Geometry: final body of the model. Coordinates: model frame, mm. Coordinates: 2 decimals unless noted, no trailing zeros. Write each loop counter-clockwise with the first axis right and the second up, starting at its lowest first coordinate (ties: lowest second). Pieces come first, ordered by that corner, then holes. Notation, with made-up numbers: (30, 3.25) - (66, 3.25) arc R33 ccw to (66, 40.25) - close; hole circle Ø11 at (-39.75, -13). An arc over 180 degrees is marked (long way). Put each result on its own line as item: value.
```python
from build123d import *

# Parameters (mm, degrees)
ESQUISSE1_W                = 381
ESQUISSE1_H                = 381
BOSS_EXTRU_1_DEPTH         = 6.35
ESQUISSE2_W                = 38.1
ESQUISSE2_H                = 6.35
BOSS_EXTRU_2_DEPTH         = 6.35
R_P_TITION_LIN_AIRE1_COUNT = 4
R_P_TITION_LIN_AIRE1_PITCH = 76.2
SYM_TRIE1_COPY_1_SKETCH_W  = 38.1
SYM_TRIE1_COPY_1_SKETCH_H  = 6.35
SYM_TRIE1_COPY_1_DEPTH     = 6.35
SYM_TRIE1_COPY_2_SKETCH_W  = 38.1
SYM_TRIE1_COPY_2_SKETCH_H  = 6.35
SYM_TRIE1_COPY_2_DEPTH     = 6.35
SYM_TRIE1_COPY_3_SKETCH_W  = 38.1
SYM_TRIE1_COPY_3_SKETCH_H  = 6.35
SYM_TRIE1_COPY_3_DEPTH     = 6.35
ESQUISSE3_W                = 38.1
ESQUISSE3_H                = 6.35
BOSS_EXTRU_3_DEPTH         = 6.35
R_P_TITION_LIN_AIRE2_COUNT = 4
R_P_TITION_LIN_AIRE2_PITCH = 76.2
SYM_TRIE2_COPY_1_SKETCH_W  = 38.1
SYM_TRIE2_COPY_1_SKETCH_H  = 6.35
SYM_TRIE2_COPY_1_DEPTH     = 6.35
SYM_TRIE2_COPY_2_SKETCH_W  = 38.1
SYM_TRIE2_COPY_2_SKETCH_H  = 6.35
SYM_TRIE2_COPY_2_DEPTH     = 6.35
SYM_TRIE2_COPY_3_SKETCH_W  = 38.1
SYM_TRIE2_COPY_3_SKETCH_H  = 6.35
SYM_TRIE2_COPY_3_DEPTH     = 6.35


with BuildPart() as part:
    # Esquisse1 → Boss.-Extru.1 (new body)
    with BuildSketch(Plane(origin=(0, 0, 0), x_dir=(1, 0, 0), z_dir=(0, 1, 0))):
        Rectangle(ESQUISSE1_W, ESQUISSE1_H)
    extrude(amount=BOSS_EXTRU_1_DEPTH)

    # Esquisse2 → Boss.-Extru.2 (add)
    with BuildSketch(Plane(origin=(190.5, 0, 0), x_dir=(0, 0, -1), z_dir=(1, 0, 0))):
        with Locations((-114.3, 3.175)):
            Rectangle(ESQUISSE2_W, ESQUISSE2_H)
    boss_extru_2 = extrude(amount=BOSS_EXTRU_2_DEPTH)

    # Répétition linéaire1: Boss.-Extru.2 ×4
    with Locations(*[(0, 0, -i * R_P_TITION_LIN_AIRE1_PITCH) for i in range(1, R_P_TITION_LIN_AIRE1_COUNT)]):
        add(boss_extru_2)

    # Symétrie1: Boss.-Extru.2 across plane
    add(boss_extru_2.mirror(Plane(origin=(0, 0, 0), x_dir=(0, 0, 1), z_dir=(1, 0, 0))))

    # Symétrie1 copy 1 sketch → Symétrie1 copy 1 (add)
    with BuildSketch(Plane(origin=(-190.5, 0, -76.2), x_dir=(0, 0, -1), z_dir=(-1, 0, 0))):
        with Locations((-114.3, -3.175)):
            Rectangle(SYM_TRIE1_COPY_1_SKETCH_W, SYM_TRIE1_COPY_1_SKETCH_H)
    extrude(amount=SYM_TRIE1_COPY_1_DEPTH)

    # Symétrie1 copy 2 sketch → Symétrie1 copy 2 (add)
    with BuildSketch(Plane(origin=(-190.5, 0, -152.4), x_dir=(0, 0, -1), z_dir=(-1, 0, 0))):
        with Locations((-114.3, -3.175)):
            Rectangle(SYM_TRIE1_COPY_2_SKETCH_W, SYM_TRIE1_COPY_2_SKETCH_H)
    extrude(amount=SYM_TRIE1_COPY_2_DEPTH)

    # Symétrie1 copy 3 sketch → Symétrie1 copy 3 (add)
    with BuildSketch(Plane(origin=(-190.5, 0, -228.6), x_dir=(0, 0, -1), z_dir=(-1, 0, 0))):
        with Locations((-114.3, -3.175)):
            Rectangle(SYM_TRIE1_COPY_3_SKETCH_W, SYM_TRIE1_COPY_3_SKETCH_H)
    extrude(amount=SYM_TRIE1_COPY_3_DEPTH)

    # Esquisse3 → Boss.-Extru.3 (add)
    with BuildSketch(Plane.XY.offset(190.5)):
        with Locations((114.3, 3.175)):
            Rectangle(ESQUISSE3_W, ESQUISSE3_H)
    boss_extru_3 = extrude(amount=BOSS_EXTRU_3_DEPTH)

    # Répétition linéaire2: Boss.-Extru.3 ×4
    with Locations(*[(-i * R_P_TITION_LIN_AIRE2_PITCH, 0, 0) for i in range(1, R_P_TITION_LIN_AIRE2_COUNT)]):
        add(boss_extru_3)

    # Symétrie2: Boss.-Extru.3 across plane
    add(boss_extru_3.mirror(Plane.XY))

    # Symétrie2 copy 1 sketch → Symétrie2 copy 1 (add)
    with BuildSketch(Plane(origin=(-76.2, 0, -190.5), x_dir=(1, 0, 0), z_dir=(0, 0, -1))):
        with Locations((114.3, -3.175)):
            Rectangle(SYM_TRIE2_COPY_1_SKETCH_W, SYM_TRIE2_COPY_1_SKETCH_H)
    extrude(amount=SYM_TRIE2_COPY_1_DEPTH)

    # Symétrie2 copy 2 sketch → Symétrie2 copy 2 (add)
    with BuildSketch(Plane(origin=(-152.4, 0, -190.5), x_dir=(1, 0, 0), z_dir=(0, 0, -1))):
        with Locations((114.3, -3.175)):
            Rectangle(SYM_TRIE2_COPY_2_SKETCH_W, SYM_TRIE2_COPY_2_SKETCH_H)
    extrude(amount=SYM_TRIE2_COPY_2_DEPTH)

    # Symétrie2 copy 3 sketch → Symétrie2 copy 3 (add)
    with BuildSketch(Plane(origin=(-228.6, 0, -190.5), x_dir=(1, 0, 0), z_dir=(0, 0, -1))):
        with Locations((114.3, -3.175)):
            Rectangle(SYM_TRIE2_COPY_3_SKETCH_W, SYM_TRIE2_COPY_3_SKETCH_H)
    extrude(amount=SYM_TRIE2_COPY_3_DEPTH)


solid = part.part
```
1. Section query B-B (x = 149.5). Return loops of the section in (y, z).
Answer below:
outline: (0, -190.5) - (6.35, -190.5) - (6.35, 190.5) - (0, 190.5) - close
2. Ray query, probe 1 along Z at (x, y) = (-4, 1.75). Return the intervals inside material, ascending. Write a range as from..to.
Answer below:
probe 1: z = -190.5..190.5
3. Section query A-A (z = -167). Return loops of the section in (x, y).
Answer below:
outline: (-190.5, 0) - (190.5, 0) - (190.5, 6.35) - (-190.5, 6.35) - close
4. Pin query (flat end, axial travel): pin 1 Ø1.5 at (x, y) = (-1.5, 4.5) entering from +Z; pin 2 Ø1.9 at (y, z) = (1.5, 194) entering from +X; pin 3 Ø1.9 at (x, y) = (193.5, 2.5) entering from +Z. Return the tip coordinate at first contact, or that it passes through.
Answer below:
pin 1: stops at z = 190.5
pin 2: stops at x = 133.35
pin 3: stops at z = 133.35
